Can you work these out from the model? Positions are in its coordinate system, mm. A direction names the side the tool comes from. Coordinates: 2 decimals unless noted, no trailing zeros. Order: outer loops, then holes, each group sorted by start corner. A loop starts at its lowest first (then second) coordinate and runs counter-clockwise, first axis right, second up.
```python
from build123d import *

# Parameters (mm, degrees)
BOSS_EXTRUDE1_DEPTH = 701.675
SHELL1_T            = -12.7
SKETCH3_W           = 49.6
SKETCH3_H           = 290
CUT_EXTRUDE1_DEPTH  = 20
BOSS_EXTRUDE2_REACH = 980.494
CHAMFER1_SIZE       = 12.7
CHAMFER1_SIZE_2     = 20


with BuildPart() as part:
    # Sketch2 → Boss-Extrude1 (new, symmetric)
    with BuildSketch(Plane.XY):
        Polygon((0, 0), (-125, 216.506350946), (-532.280287957, 356.869859221), (75, 410), (75, -240), (0, -240), align=None)
    extrude(amount=BOSS_EXTRUDE1_DEPTH, both=True)

    # Shell1
    shell1_openings = [part.faces().sort_by_distance(p)[0] for p in [
        (-228.640143978, 383.434929611, 0),
    ]]
    offset(amount=SHELL1_T, openings=shell1_openings, kind=Kind.INTERSECTION)

    # Sketch3 → Cut-Extrude1 (cut)
    with BuildSketch(Plane.XY.offset(701.675)):
        with Locations((37.5, -82.3)):
            Rectangle(SKETCH3_W, SKETCH3_H)
    extrude(amount=-CUT_EXTRUDE1_DEPTH, mode=Mode.SUBTRACT)

    # Sketch4 → Boss-Extrude2 (add, up to next)
    with BuildSketch(Plane(origin=(12.7, 0, 0), x_dir=(0, 0, -1), z_dir=(1, 0, 0)), mode=Mode.PRIVATE) as boss_extrude2_sk1:
        Polygon((688.975, -227.3), (688.975, -83.238879933), (-681.675, -227.3), align=None)
    boss_extrude2_tool1 = extrude(boss_extrude2_sk1.sketch, amount=BOSS_EXTRUDE2_REACH, mode=Mode.PRIVATE) - part.part
    add(boss_extrude2_tool1.solids().sort_by_distance((12.7, -179.279627, -232.091667))[0])

    # Chamfer1
    # the kernel refuses this chamfer: 20, 12.7 mm, written as the material it adds along each edge
    # the kernel refuses this chamfer: 20, 12.7 mm, written as the material it takes off along each edge
    with BuildSketch(Plane(origin=(12.7, -227.3, 701.675), x_dir=(0, -0.9986795899881412, 0.05137194313161755), z_dir=(1, 0, 0))) as chamfer1_2_piece_1:
        Polygon((CHAMFER1_SIZE * 0.998679589988, CHAMFER1_SIZE * 0.0513719431316), (-CHAMFER1_SIZE_2 * 0.0513719431316, CHAMFER1_SIZE_2 * 0.998679589988), (0, 0), align=None)
    extrude(amount=49.6, mode=Mode.SUBTRACT)


solid = part.part
```
1. On a 3-axis mill with a long thin cutter (end or side, diameter ignored), from which of +Z, -Z, +X, -X, +Y, -Y can I reach the whole of each face in a straight line? I mean faces 1 (the flat face through (37.15, -154.26, -13.24)), 2 (the flat face through (0, -122, 10)), 3 (the flat face through (-92, 255, 701.675)), 4 (the flat face through (-50.934, 113.62, 9.646)), 5 (the flat face through (-92, 183, -701.675)). Say none if no direction works.
Completed:
face 1: +Z, +Y
face 2: +Z, -Z, -X, -Y
face 3: +Z, +X, -X, +Y, -Y
face 4: +Y
face 5: -Z, +X, -X, +Y, -Y
2. Imagine slicing it at D-D on z = 532.5. Please give me the cut outline in (x, y).
Completed:
outline: (-532.28, 356.87) - (-125, 216.51) - (0, 0) - (0, -240) - (75, -240) - (75, 410) - (62.3, 408.89) - (62.3, -211.62) - (12.7, -211.62) - (12.7, 3.4) - (-116.37, 226.97) - (-501.19, 359.59) - close
3. Thinking about a two-plate mould opening in X: for faces 6 (the flat face through (-93, 237, -688.975)), 7 (the flat face through (38, -240, 10)), 8 (the flat face through (-325.789, 285.706, 9.823)), which applies, pulls with the +X half, pulls with the -X half, needs draft (parallel to the pull), parting line crosses it, or undercut?
Completed:
face 6: undercut
face 7: needs draft
face 8: pulls with the -X half
4. Please list where these lines run through material, in increasing order: probe 1 along X at (y, z) = (-169, 556.5); probe 2 along Z at (x, y) = (-51, 216) (3 decimals); probe 3 along Y at (x, z) = (-435.5, -452).
Completed:
probe 1: x = 0 to 12.7, 62.3 to 75
probe 2: z = -701.675 to -688.975, 688.975 to 701.675
probe 3: y = 323.52 to 336.95
5. I'm going to push flat-ended pins straight in: pin 1 (5 mm diameter, centred on x = -116, z = -405.5, fed in from -Y); pin 2 (1 mm diameter, centred on x = -369, z = -427.5, fed in from -Y); pin 3 (12 mm diameter, centred on y = -78.5, z = 269, fed in from -X). Where does each tip first touch, or does it pass through?
Completed:
pin 1: stops at y = 196.59
pin 2: stops at y = 300.43
pin 3: stops at x = 0
6. Imagine slicing it at C-C on z = -499.5. Please give me the cut outline in (x, y).
Completed:
outline: (-532.28, 356.87) - (-125, 216.51) - (0, 0) - (0, -240) - (75, -240) - (75, 410) - (62.3, 408.89) - (62.3, -103.15) - (12.7, -103.15) - (12.7, 3.4) - (-116.37, 226.97) - (-501.19, 359.59) - close
7. Imagine slicing it at A-A on y = -63.5. Please give me the cut outline in (x, z) (3 decimals), then the cut area to 3 significant figures.
Completed:
outline: (0, -701.675) - (75, -701.675) - (75, 701.675) - (62.3, 701.675) - (62.3, -688.975) - (12.7, -688.975) - (12.7, 701.675) - (0, 701.675) - close
area: 36,300 mm2
8. Imagine slicing it at B-B on x = -442.5. Please give me the cut outline in (y, z) (3 decimals), then the cut area to 3 significant figures.
Completed:
outline: (325.928, -701.675) - (364.725, -701.675) - (364.725, -688.975) - (339.361, -688.975) - (339.361, 688.975) - (364.725, 688.975) - (364.725, 701.675) - (325.928, 701.675) - close
area: 19,500 mm2
